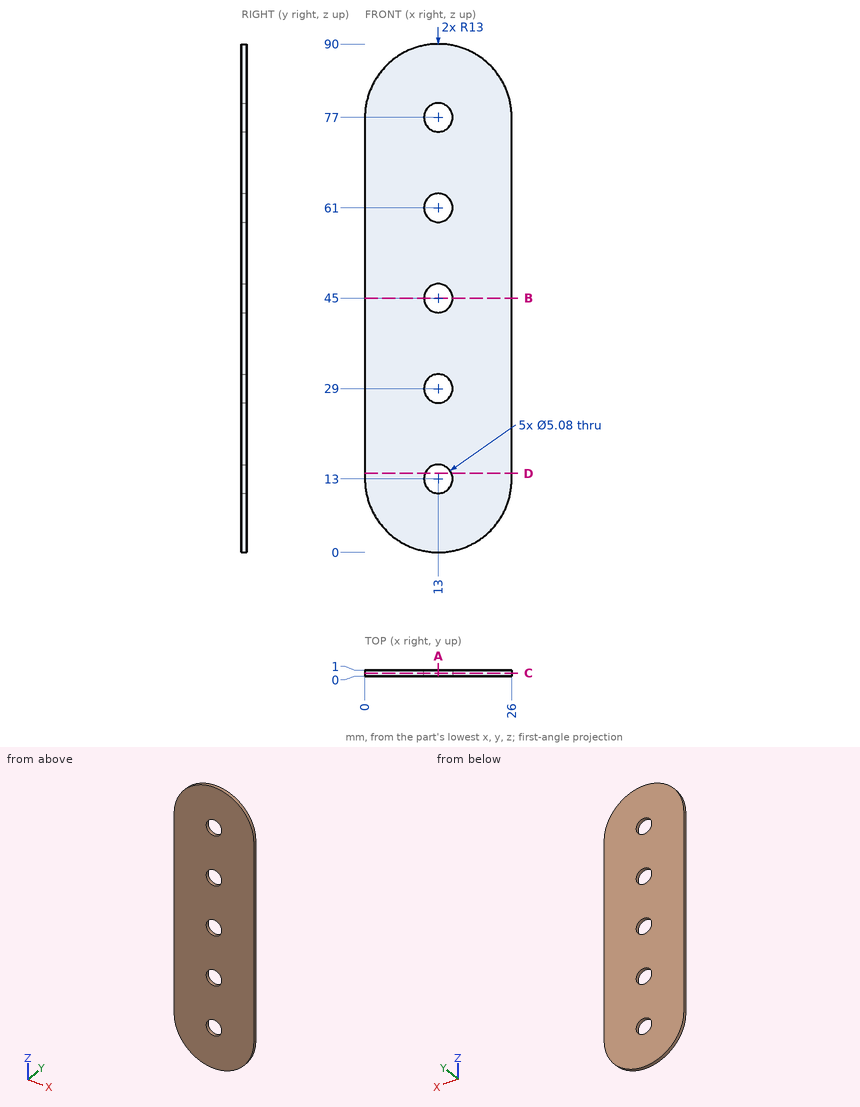
Answer from the drawing. Dimensions are ordinates in mm from the lowest x, y and z of the part. Give positions to 0.01 mm unless a question says otherwise; leave off trailing zeros. Write each loop counter-clockwise with the first axis right and the second up, starting at its lowest first coordinate (ties: lowest second). Pieces come first, ordered by that corner, then holes.
1) Section C-C (y = 0.5) is taken. Write down the section's boundary in (x, z), and give its area (3 significant figures).
2) Section A-A (x = 13) is taken. Write down the section's boundary in (y, z), and give its area (3 significant figures).
3) Section B-B (z = 45) is taken. Write down the section's boundary in (x, y), and give its area (3 significant figures).
4) Find the intervals of material crossed by L1, parallel to Z at x = 13, y = 0.55; L2, parallel to Z at x = 12, y = 0.45; L3, parallel to X at y = 0.9, z = 12, in increasing order.
5) Section D-D (z = 14) is taken. Write down the section's boundary in (x, y), and give its area (3 significant figures).
Response:
1. outline: (0, 13) arc R13 ccw to (26, 13) - (26, 77) arc R13 ccw to (0, 77) - close; hole circle Ø5.08 at (13, 13); hole circle Ø5.08 at (13, 29); hole circle Ø5.08 at (13, 45); hole circle Ø5.08 at (13, 61); hole circle Ø5.08 at (13, 77)
1. area: 2,090 mm2
2. outline: (0, 0) - (1, 0) - (1, 10.46) - (0, 10.46) - close; (0, 15.54) - (1, 15.54) - (1, 26.46) - (0, 26.46) - close; (0, 31.54) - (1, 31.54) - (1, 42.46) - (0, 42.46) - close; (0, 47.54) - (1, 47.54) - (1, 58.46) - (0, 58.46) - close; (0, 63.54) - (1, 63.54) - (1, 74.46) - (0, 74.46) - close; (0, 79.54) - (1, 79.54) - (1, 90) - (0, 90) - close
2. area: 64.6 mm2
3. outline: (0, 0) - (10.46, 0) - (10.46, 1) - (0, 1) - close; (15.54, 0) - (26, 0) - (26, 1) - (15.54, 1) - close
3. area: 20.9 mm2
4. L1: z = 0 to 10.46, 15.54 to 26.46, 31.54 to 42.46, 47.54 to 58.46, 63.54 to 74.46, 79.54 to 90
4. L2: z = 0.04 to 10.67, 15.33 to 26.67, 31.33 to 42.67, 47.33 to 58.67, 63.33 to 74.67, 79.33 to 89.96
4. L3: x = 0.04 to 10.67, 15.33 to 25.96
5. outline: (0, 0) - (10.67, 0) - (10.67, 1) - (0, 1) - close; (15.33, 0) - (26, 0) - (26, 1) - (15.33, 1) - close
5. area: 21.3 mm2
